Study the drawing (mm; zero at the part's minimum x, y, z) and answer. Coordinates: 2 decimals unless noted, no trailing zeros. Order: outer loops, then holes, each group sorted by start corner. A loop starts at its lowest first (then second) coordinate and runs counter-clockwise, first axis right, second up. Notation, with made-up numbers: M -10,74.5 L 28,74.5 A23 ccw 28,83.5 Z; hole C -39.5,63.25 d10. An arc over 180 degrees is marked long. Use a Markdown table: item, result. Add a question column.
1) Find section A-A on z = 0.95. Write down the section's boundary in (x, y).
2) Find section B-B on y = 34. Write down the section's boundary in (x, z).
3) This flat-tipped pin is pushed along its axis until it touches: pin 1 Ø0.8 at (y, z) = (17, 1) entering from +X. Where does it stop, or does it pass through?
4) Find the intervals of material crossed by probe 1 along Y at (x, z) = (19.5, 1); probe 2 along Y at (x, z) = (20, 1); probe 3 along X at (y, z) = (84, 0.8), in increasing order. Write a range as [from, to].
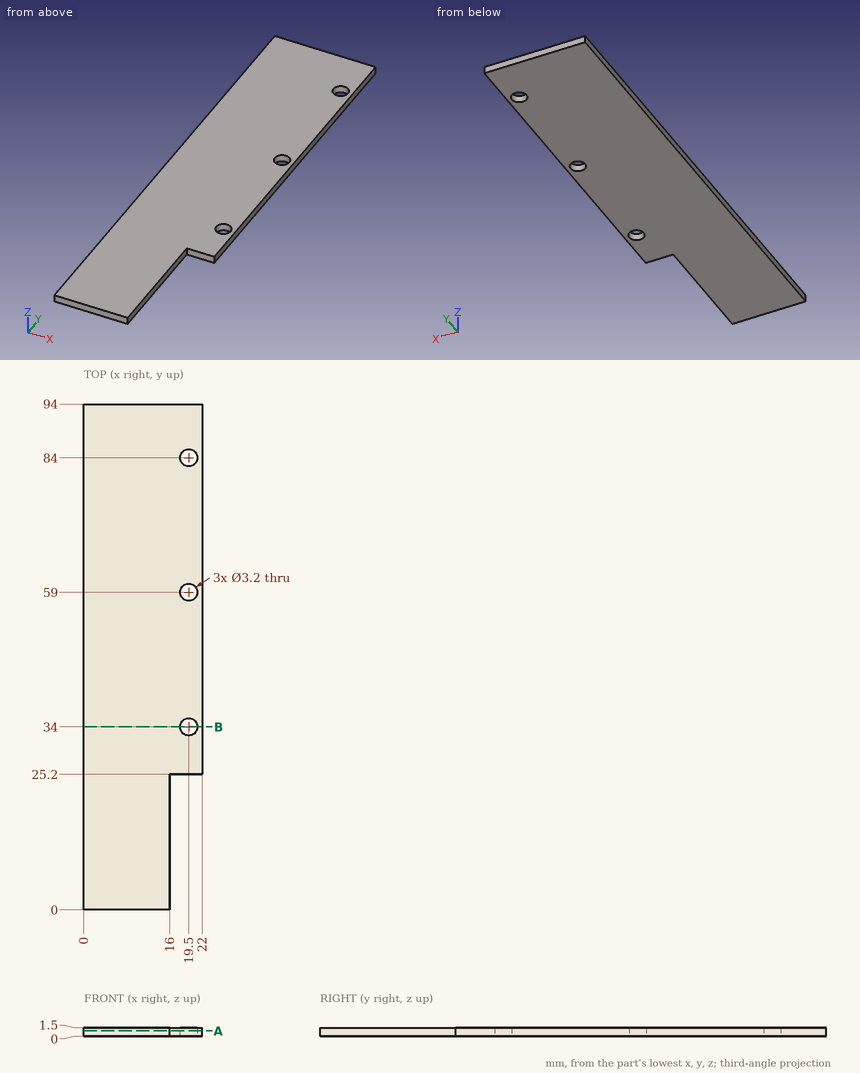
Check result:
| question | item | result |
|---|---|---|
| 1 | outline | M 0,0 L 16,0 L 16,25.2 L 22,25.2 L 22,94 L 0,94 Z; hole C 19.5,34 d3.2; hole C 19.5,59 d3.2; hole C 19.5,84 d3.2 |
| 2 | outline | M 0,0 L 17.9,0 L 17.9,1.5 L 0,1.5 Z; M 21.1,0 L 22,0 L 22,1.5 L 21.1,1.5 Z |
| 3 | pin 1 | stops at x = 16 |
| 4 | probe 1 | y = [25.2, 32.4], [35.6, 57.4], [60.6, 82.4], [85.6, 94] |
| 4 | probe 2 | y = [25.2, 32.48], [35.52, 57.48], [60.52, 82.48], [85.52, 94] |
| 4 | probe 3 | x = [0, 17.9], [21.1, 22] |
